Read the model definition and answer for the solid it produces. Units are mm, in the model's axes. Face numbers are marked on the shaded views. A direction names the side the tool comes from. Give positions to 0.01 mm unless a question says otherwise; leave off trailing zeros. Loops run counter-clockwise (first coordinate to the right, second up) from the corner with the lowest first, then second, coordinate; pieces in that order, holes last. Notation, with made-up numbers: (42.5, 35.25) - (60.5, 35.25) arc R27 ccw to (60.5, 52.25) - close; hole circle Ø9 at (58, 50). An arc over 180 degrees is marked (long way). Put each result on its own line as item: value. Start each with the question number.
1. Given pin 1 Ø3 at (x, y) = (1.5, -6) entering from -Z; pin 2 Ø1.5 at (x, y) = (2, 4.5) entering from -Z; pin 3 Ø1 at (x, y) = (2, 2) entering from +Z, each flat-ended and moving along its own axis, determine where each tip first touches the part or whether it passes through.
2. A cutting plane is placed at C-C, the plane x = 1.55. Determine the outline of the cut face in (y, z), plus the area to 3 significant figures.
3. For the marked faces 3 and 4, determine the directions among +Z, -Z, +X, -X, +Y, -Y from which every point of the face is accessible in a straight line to the end or side of a thin tool.
4. Consider L1, parallel to Z at x = 0.45, y = 0; L2, parallel to Z at x = 1.8, y = 0; L3, parallel to Z at x = 1.4, y = -1. Determine where each line is inside the solid, lowest interval first. Write a range as from..to.
5. For a pull along Y with two mould halves and no side action, classify the marked faces 1 and 2 as released by +Y, released by -Y, zero draft, split by the parting line, or undercut.
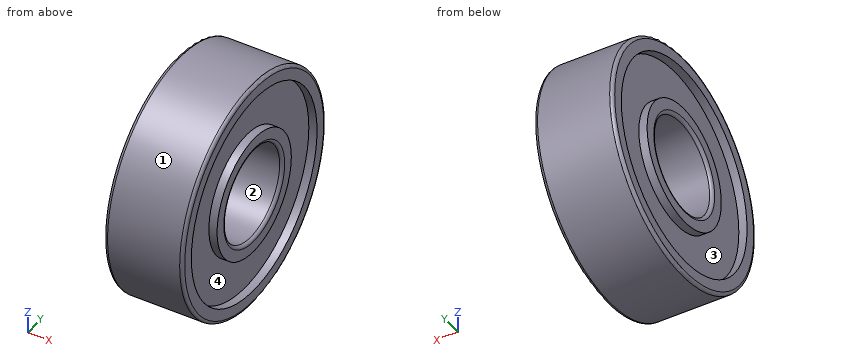
```python
from build123d import *


with BuildPart() as part:
    # Sketch1 → Revolve1 (revolve)
    with BuildSketch(Plane.XY):
        with BuildLine():
            Line((0, 3.9), (0, 3.2))
            ThreePointArc((0, 3.2), (0.058578644, 3.058578644), (0.2, 3))
            Line((0.2, 3), (4.8, 3))
            ThreePointArc((4.8, 3), (4.941421356, 3.058578644), (5, 3.2))
            Line((5, 3.2), (5, 3.9))
            Line((5, 3.9), (4.4765, 3.9))
            Line((4.4765, 3.9), (4.4765, 6.6))
            Line((4.4765, 6.6), (5, 6.6))
            Line((5, 6.6), (5, 7.3))
            ThreePointArc((5, 7.3), (4.941421356, 7.441421356), (4.8, 7.5))
            Line((4.8, 7.5), (0.2, 7.5))
            ThreePointArc((0.2, 7.5), (0.058578644, 7.441421356), (0, 7.3))
            Line((0, 7.3), (0, 6.6))
            Line((0, 6.6), (0.5235, 6.6))
            Line((0.5235, 6.6), (0.5235, 3.9))
            Line((0.5235, 3.9), (0, 3.9))
        make_face()
    revolve(axis=Axis((-0.001349798, 0, 0), (1, 0, 0)))


solid = part.part
```
Return value:
1. pin 1: stops at z = -6
1. pin 2: stops at z = -6.5
1. pin 3: stops at z = 7.35
2. outline: circle Ø15 at (0, 0); hole circle Ø6 at (0, 0)
2. area: 148 mm2
3. face 3: -X
3. face 4: +X
4. L1: z = -7.5..-6.6, -3.9..-3, 3..3.9, 6.6..7.5
4. L2: z = -7.5..-3, 3..7.5
4. L3: z = -7.43..-2.83, 2.83..7.43
5. face 1: split by the parting line
5. face 2: undercut
